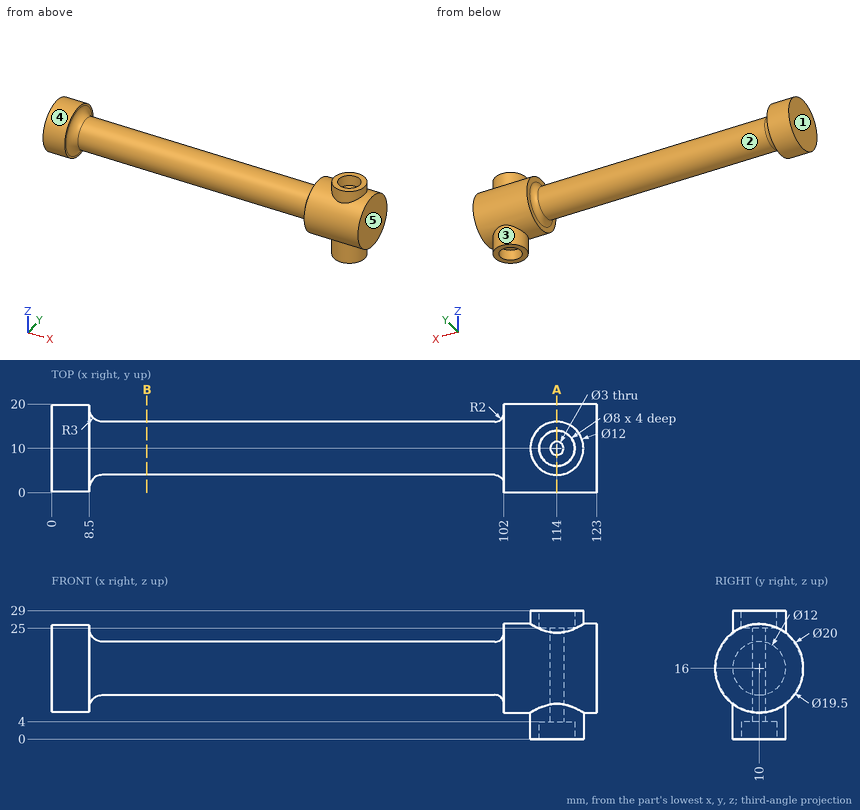
Check sheet for the drawn part. Datum: minimum x, y, z corner. Units: mm. A direction names the side the tool comes from. Coordinates: 2 decimals unless noted, no trailing zeros. Loops run counter-clockwise (first coordinate to the right, second up) from the corner with the lowest first, then second, coordinate; pieces in that order, holes last. Notation, with made-up numbers: (34, 43) -> (75, 43) arc R28 cw to (75, 82) -> close; hole circle Ø4 at (57.5, -35.75). An arc over 180 degrees is marked (long way). Answer in a Markdown table with one row per item.
1) Access from +Z, -Z, +X, -X, +Y, -Y to the whole of each face (thin tool, end or side, straight path). Record for the marked faces 4 and 5.
The answers:
| item | result |
|---|---|
| face 4 | -X |
| face 5 | +Z, -Z, +X, +Y, -Y |
2) Section check B-B (x = 21.5). Record the cut outline in (y, z).
The answers:
| item | result |
|---|---|
| outline | circle Ø12 at (10, 16) |
3) Section check A-A (x = 114). Record the cut outline in (y, z).
The answers:
| item | result |
|---|---|
| outline | (4, 0) -> (6, 0) -> (6, 4) -> (8.5, 4) -> (8.5, 25) -> (6, 25) -> (6, 29) -> (4, 29) -> (4, 24) arc R10 ccw to (4, 8) -> close; (11.5, 4) -> (14, 4) -> (14, 0) -> (16, 0) -> (16, 8) arc R10 ccw to (16, 24) -> (16, 29) -> (14, 29) -> (14, 25) -> (11.5, 25) -> close |
4) Scan lines: line 1 along X through (y, z) = (1, 15.25); line 2 along Y through (x, z) = (114, 2.7); line 3 along Y through (x, z) = (114, 19.5). Record each from-to range of solid material in increasing order. Write a range as from..to.
The answers:
| item | result |
|---|---|
| line 1 | x = 0..8.5, 102..123 |
| line 2 | y = 4..6, 14..16 |
| line 3 | y = 0.63..8.5, 11.5..19.37 |
5) Draft check along X on the marked faces 1, 2 and 3. Enter one of: released by +X, released by -X, zero draft, split by the parting line, or undercut.
The answers:
| item | result |
|---|---|
| face 1 | released by -X |
| face 2 | undercut |
| face 3 | split by the parting line |
6) Depth check by flat-ended pin: P1, Ø9, axis at x = 116, y = 10, coming from the -Z side; P2, Ø4, axis at x = 106.5, y = 4, coming from the -Z side; P3, Ø4, axis at x = 31.5, y = 15, coming from the -Z side; P4, Ø2, axis at x = 86, y = 12, coming from the +Z side. Enter the tip coordinate at first touch or a pass-through.
The answers:
| item | result |
|---|---|
| P1 | stops at z = 0 |
| P2 | stops at z = 6.83 |
| P3 | stops at z = 10.8 |
| P4 | stops at z = 21.92 |
